For this review, take the finished solid that the model builds, in its own axes (mm). A direction names the side the tool comes from. Round coordinates to 2 decimals unless told otherwise and drop trailing zeros. Answer in a Markdown table with one row per item.
```python
from build123d import *

# Parameters (mm, degrees)
BOSS_EXTRUDE1_DEPTH = 6.752040791
BOSS_EXTRUDE1_TAPER = 31.717474411
SKETCH3_R           = 1
CUT_EXTRUDE1_DEPTH  = 2
CIRPATTERN1_COUNT   = 5


with BuildPart() as part:
    # Sketch1 → Boss-Extrude1 (new body)
    with BuildSketch(Plane(origin=(0, 0, 0), x_dir=(1, 0, 0), z_dir=(0, 1, 0))):
        Polygon((0, 10.803265266), (-10.274515829, 3.338392562), (-6.35, -8.740025195), (6.35, -8.740025195), (10.274515829, 3.338392562), align=None)
    extrude(amount=BOSS_EXTRUDE1_DEPTH, taper=BOSS_EXTRUDE1_TAPER)

    # Sketch3 → Cut-Extrude1 (cut)
    with BuildSketch(Plane(origin=(0, 3.908658092, 6.324341644), x_dir=(1, 0, 0), z_dir=(0, 0.525731112, 0.850650808))):
        with Locations((-2, -0.626153166)):
            Circle(SKETCH3_R)
        with Locations((2, -0.626153166)):
            Circle(SKETCH3_R)
    cut_extrude1 = extrude(amount=-CUT_EXTRUDE1_DEPTH, mode=Mode.SUBTRACT)

    # CirPattern1: Cut-Extrude1 ×5 about axis
    cirpattern1_axis = Axis((0, 0, 0), (0, 1, 0))
    for i in range(1, CIRPATTERN1_COUNT):
        add(cut_extrude1.rotate(cirpattern1_axis, i * 360 / CIRPATTERN1_COUNT), mode=Mode.SUBTRACT)


solid = part.part
```
Q1. For probe 1 along X at (y, z) = (2, 4); probe 2 along Y at (x, z) = (-5, 4); probe 3 along Z at (x, y) = (-2, 5.75), list the stretches that pass through material, from the lowest coordinate up.
Found:
| item | result |
|---|---|
| probe 1 | -6.59 to -5.33, -4.12 to 4.12, 5.33 to 6.59 |
| probe 2 | 0 to 1.83, 4.1 to 4.45 |
| probe 3 | -4.96 to 5.19 |
Q2. Insertion check: P1, Ø1, axis at x = -5, z = 3.5, coming from the -Y side; P2, Ø4, axis at y = 1.5, z = 1.5, coming from the +X side; P3, Ø4, axis at x = 2.5, y = 1, coming from the +Z side; P4, Ø3, axis at x = -4, y = 5.5, coming from the -Z side. Each pin has a flat end and moves straight along its axis. Give the tip position at first contact, or say it passes through.
Found:
| item | result |
|---|---|
| P1 | y = 0 |
| P2 | x = 9.13 |
| P3 | z = 8.74 |
| P4 | z = -5.28 |
Q3. Machinability: for faces 4 (the face through (-5.325, 2.336, -0.387)), 5 (the face through (0, 6.752, 0)), which of the approach directions +Z, -Z, +X, -X, +Y, -Y give a long, thin tool a straight path to every point of the face, cutting with its end or side? Answer none if there is none.
Found:
| item | result |
|---|---|
| face 4 | none |
| face 5 | +Z, -Z, +X, -X, +Y |
Q4. Take a section at A-A (z = -3). State how many separate pieces and enclosed holes the cut face has, then the cut area to 3 significant figures.
Found:
| item | result |
|---|---|
| separate pieces | 1 |
| enclosed holes | 2 |
| area | 90.4 mm² |
Q5. Mouldability with a two-part tool opening along X and no side actions: class faces 1 (the face through (1.986, 2.336, 4.945)), 2 (the face through (5.389, 2.532, 2.883)), 3 (the face through (-1, 0, 0)) as +X half, -X half, draft (parallel to the pull), parting line (faces both ways), or undercut.
Found:
| item | result |
|---|---|
| face 1 | undercut |
| face 2 | undercut |
| face 3 | draft |
